Autodesk Inventor part; units mm, degrees
ref_plane "s1_XY" through (25.4, 0, 19.05) normal (1, 0, 0) x (0, 0, -1)
ref_plane "s1_YZ" through (25.4, 0, 19.05) normal (0, 0, -1) x (0, 1, 0)
ref_plane "s1_ZX" through (25.4, 0, 19.05) normal (0, 1, 0) x (1, 0, 0)
sketch "Sketch_1" plane through (0, 0, 0) normal (0, 0, 1) x (1, 0, 0)
  line L0 (-15.875, -25.4) -> (-15.875, -31.75)
  line L1 (-15.875, -31.75) -> (21.59, -31.75)
  line L2 (21.59, -31.75) -> (22.225, -32.385)
  line L3 (22.225, -32.385) -> (22.225, -50.165)
  line L4 (22.225, -50.165) -> (22.86, -50.8)
  line L5 (22.86, -50.8) -> (31.115, -50.8)
  line L6 (31.115, -50.8) -> (31.75, -50.165)
  line L7 (31.75, -50.165) -> (31.75, 50.165)
  line L8 (31.75, 50.165) -> (31.115, 50.8)
  line L9 (31.115, 50.8) -> (22.86, 50.8)
  line L10 (22.86, 50.8) -> (22.225, 50.165)
  line L11 (22.225, 50.165) -> (22.225, 32.385)
  line L12 (22.225, 32.385) -> (21.59, 31.75)
  line L13 (21.59, 31.75) -> (-15.875, 31.75)
  line L14 (-15.875, 31.75) -> (-15.875, 25.4)
  line L15 (-15.875, 25.4) -> (19.05, 25.4)
  line L16 (19.05, 25.4) -> (25.4, 19.05)
  line L17 (25.4, 19.05) -> (25.4, -19.05)
  line L18 (25.4, -19.05) -> (19.05, -25.4)
  line L19 (19.05, -25.4) -> (-15.875, -25.4)
extrude "Extrusion1" add sketch "Sketch_1" along normal mid plane 71.4248
sketch "Sketch2" plane through (31.75, -50.165, 35.7124) normal (1, 0, 0) x (0, 0, -1)
  point P0 (16.6624, 91.44)
hole "Hole1" at (31.75, 41.275, 19.05) direction (-1, 0, 0) diameter 8.3312 depth 9.525
pattern_linear "Rectangular Pattern1" count 2 spacing 38.1 along (0, 0, -1) count 2 spacing 82.55 along (0, -1, 0) of "Hole1"
sketch "Sketch3" plane through (31.75, -50.165, 35.7124) normal (1, 0, 0) x (0, 0, -1)
  point P0 (16.6624, 50.165)
hole "Hole2" at (31.75, 0, 19.05) direction (-1, 0, 0) diameter 5.1054 depth 6.35 countersink diameter 9.779 countersink angle 100
pattern_linear "Rectangular Pattern2" count 2 spacing 38.1 along (0, 0, -1) of "Hole2"
sketch "Sketch4" plane through (-15.875, 31.75, 35.7124) normal (0, 1, 0) x (1, 0, 0)
  point P0 (15.875, 16.6624)
hole "Hole3" at (0, 31.75, 19.05) direction (0, -1, 0) diameter 5.1054 depth 6.35 countersink diameter 9.779 countersink angle 100
pattern_linear "Rectangular Pattern3" count 2 spacing 38.1 along (0, 0, -1) of "Hole3"
sketch "Sketch5" plane through (-15.875, -31.75, 35.7124) normal (0, -1, 0) x (1, 0, 0)
  point P0 (15.875, -16.6624)
hole "Hole4" at (0, -31.75, 19.05) direction (0, 1, 0) diameter 5.1054 depth 6.35 countersink diameter 9.779 countersink angle 100
pattern_linear "Rectangular Pattern4" count 2 spacing 38.1 along (0, 0, -1) of "Hole4"
ref_plane "s1_XY" through (25.4, 0, 19.05) normal (1, 0, 0) x (0, 0, -1)
ref_plane "s1_YZ" through (25.4, 0, 19.05) normal (0, 0, -1) x (0, 1, 0)
ref_plane "s1_ZX" through (25.4, 0, 19.05) normal (0, 1, 0) x (1, 0, 0)
ref_plane "s1_2_XY" through (25.4, 0, -19.05) normal (1, 0, 0) x (0, 0, -1)
ref_plane "s1_2_YZ" through (25.4, 0, -19.05) normal (0, 0, -1) x (0, 1, 0)
ref_plane "s1_2_ZX" through (25.4, 0, -19.05) normal (0, 1, 0) x (1, 0, 0)
ref_plane "s2_XY" through (0, 25.4, 19.05) normal (0, 1, 0) x (1, 0, 0)
ref_plane "s2_YZ" through (0, 25.4, 19.05) normal (1, 0, 0) x (0, 0, -1)
ref_plane "s2_ZX" through (0, 25.4, 19.05) normal (0, 0, -1) x (0, 1, 0)
ref_plane "s2_2_XY" through (0, 25.4, -19.05) normal (0, 1, 0) x (1, 0, 0)
ref_plane "s2_2_YZ" through (0, 25.4, -19.05) normal (1, 0, 0) x (0, 0, -1)
ref_plane "s2_2_ZX" through (0, 25.4, -19.05) normal (0, 0, -1) x (0, 1, 0)
ref_plane "s3_XY" through (0, -25.4, 19.05) normal (0, 1, 0) x (1, 0, 0)
ref_plane "s3_YZ" through (0, -25.4, 19.05) normal (1, 0, 0) x (0, 0, -1)
ref_plane "s3_ZX" through (0, -25.4, 19.05) normal (0, 0, -1) x (0, 1, 0)
ref_plane "s3_2_XY" through (0, -25.4, -19.05) normal (0, 1, 0) x (1, 0, 0)
ref_plane "s3_2_YZ" through (0, -25.4, -19.05) normal (1, 0, 0) x (0, 0, -1)
ref_plane "s3_2_ZX" through (0, -25.4, -19.05) normal (0, 0, -1) x (0, 1, 0)
ref_plane "t1_1_XY" through (29.7892, 0, 19.05) normal (1, 0, 0) x (0, 0, -1)
ref_plane "t1_1_YZ" through (29.7892, 0, 19.05) normal (0, 0, -1) x (0, 1, 0)
ref_plane "t1_1_ZX" through (29.7892, 0, 19.05) normal (0, 1, 0) x (1, 0, 0)
ref_plane "t1_2_XY" through (29.7892, 0, -19.05) normal (1, 0, 0) x (0, 0, -1)
ref_plane "t1_2_YZ" through (29.7892, 0, -19.05) normal (0, 0, -1) x (0, 1, 0)
ref_plane "t1_2_ZX" through (29.7892, 0, -19.05) normal (0, 1, 0) x (1, 0, 0)
ref_plane "t2_1_XY" through (0, 29.7892, 19.05) normal (0, 1, 0) x (1, 0, 0)
ref_plane "t2_1_YZ" through (0, 29.7892, 19.05) normal (1, 0, 0) x (0, 0, -1)
ref_plane "t2_1_ZX" through (0, 29.7892, 19.05) normal (0, 0, -1) x (0, 1, 0)
ref_plane "t2_2_XY" through (0, 29.7892, -19.05) normal (0, 1, 0) x (1, 0, 0)
ref_plane "t2_2_YZ" through (0, 29.7892, -19.05) normal (1, 0, 0) x (0, 0, -1)
ref_plane "t2_2_ZX" through (0, 29.7892, -19.05) normal (0, 0, -1) x (0, 1, 0)
ref_plane "t3_1_XY" through (0, -29.7892, 19.05) normal (0, 1, 0) x (1, 0, 0)
ref_plane "t3_1_YZ" through (0, -29.7892, 19.05) normal (1, 0, 0) x (0, 0, -1)
ref_plane "t3_1_ZX" through (0, -29.7892, 19.05) normal (0, 0, -1) x (0, 1, 0)
ref_plane "t3_2_XY" through (0, -29.7892, -19.05) normal (0, 1, 0) x (1, 0, 0)
ref_plane "t3_2_YZ" through (0, -29.7892, -19.05) normal (1, 0, 0) x (0, 0, -1)
ref_plane "t3_2_ZX" through (0, -29.7892, -19.05) normal (0, 0, -1) x (0, 1, 0)
properties part number "6825_p"
Source: CAD feature listing. Evaluate the final solid. Frame: model axes, mm. A direction names the side the tool comes from. Round coordinates to 2 decimals unless told otherwise and drop trailing zeros. Loops run counter-clockwise (first coordinate to the right, second up) from the corner with the lowest first, then second, coordinate; pieces in that order, holes last. Notation, with made-up numbers: (-2.75, 70) -> (46.25, 70) arc R21 cw to (46.25, 84) -> close; hole circle Ø3 at (28.5, 42). An arc over 180 degrees is marked (long way). Answer as a JSON object with one key per item and string values. Group by question number.
Q1. Access query for faces 1 (the flat face through (1, 25.4, 0)), 2 (the flat face through (3, 31.75, 0)), 3 (the flat face through (-15.875, -29, 0)). Directions: +Z, -Z, +X, -X, +Y, -Y. A direction counts if a zero-diameter tool reaches every point of the face in a straight line with its end or side. Return the directions, or none.
Q2. Contact query for flat-ended pins moving along their axis: P1, Ø8, axis at x = 0, z = -19.05, coming from the +Y side; P2, Ø9, axis at y = -44.5, z = -11, coming from the -X side (3 decimals); P3, Ø18.5, axis at x = -5, z = 1.5, coming from the +Y side. Output: stop coordinate, or through.
Q3. Ray query, line 1 (Y direction, x = 25.75, z = 19.05); line 2 (Y direction, x = 15, z = 1); line 3 (X direction, y = -26, z = -19) (3 decimals). Return the intervals inside material, ascending. Write a range as from..to.
Q4. Mould query, pull axis Z, two halves, no side actions, for faces 4 (the flat face through (27, 0, -35.712)), 5 (the cylindrical face through (27.564, -1.725, -17.169)), 6 (the flat face through (22.225, -41, 0)), 7 (the conical face through (-1.64, -29.91, 21.19)). Classes: pulls with the +Z half, pulls with the -Z half, needs draft (parallel to the pull), parting line crosses it, or undercut.
Q5. Section query D-D (x = 14.5). Output: boundary loops of the cut face in (y, z).
Q6. Section query C-C (z = 3). Output: boundary loops of the cut face in (x, y) (3 decimals).
Q7. Section query A-A (x = 0). State how many separate pieces and enclosed holes the cut face has, plus the area to 3 significant figures.
Completed:
{
 "1": {"face 1": "+Z, -Z, -X", "face 2": "+Z, -Z, -X, +Y", "face 3": "+Z, -Z, -X, +Y, -Y"},
 "2": {"P1": "y = 31", "P2": "x = 22.225", "P3": "y = 31.75"},
 "3": {"line 1": "-50.8..-45.44, -37.11..-2.55, 2.55..37.11, 45.44..50.8", "line 2": "-31.75..-25.4, 25.4..31.75", "line 3": "-15.875..-2.552, 2.552..31.75"},
 "4": {"face 4": "pulls with the -Z half", "face 5": "undercut", "face 6": "needs draft", "face 7": "undercut"},
 "5": {"outline": "(-31.75, -35.71) -> (-25.4, -35.71) -> (-25.4, 35.71) -> (-31.75, 35.71) -> close; (25.4, -35.71) -> (31.75, -35.71) -> (31.75, 35.71) -> (25.4, 35.71) -> close"},
 "6": {"outline": "(-15.875, -31.75) -> (21.59, -31.75) -> (22.225, -32.385) -> (22.225, -50.165) -> (22.86, -50.8) -> (31.115, -50.8) -> (31.75, -50.165) -> (31.75, 50.165) -> (31.115, 50.8) -> (22.86, 50.8) -> (22.225, 50.165) -> (22.225, 32.385) -> (21.59, 31.75) -> (-15.875, 31.75) -> (-15.875, 25.4) -> (19.05, 25.4) -> (25.4, 19.05) -> (25.4, -19.05) -> (19.05, -25.4) -> (-15.875, -25.4) -> close"},
 "7": {"separate pieces": "6", "enclosed holes": "0", "area": "759 mm²"}
}
